from build123d import *

# Parameters (mm, degrees)
SKETCH1_R           = 25.5905
SKETCH1_R_2         = 19.2405
BOSS_EXTRUDE1_DEPTH = 7


with BuildPart() as part:
    # Sketch1 → Boss-Extrude1 (new body)
    with BuildSketch(Plane(origin=(0, 0, 0), x_dir=(1, 0, 0), z_dir=(0, 1, 0))):
        Circle(SKETCH1_R)
        Circle(SKETCH1_R_2, mode=Mode.SUBTRACT)
        Polygon((-12.131390351, -20.018099484), (13.231279228, -20.018099484), (13.231279228, -111.76), (38.036054145, -111.76), (38.036054145, -137.16), (-38.163945855, -137.16), (-38.163945855, -111.76), (-12.131390351, -111.76), align=None)
    extrude(amount=BOSS_EXTRUDE1_DEPTH)


solid = part.part
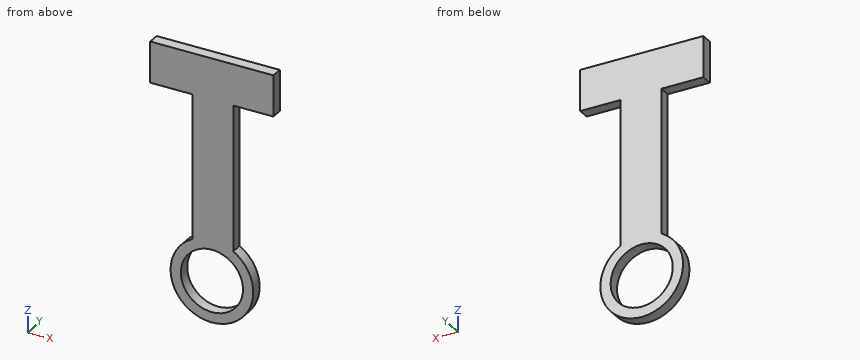
Can you work these out from the model? Positions are in its coordinate system, mm. Coordinates: 2 decimals unless noted, no trailing zeros. Loops run counter-clockwise (first coordinate to the right, second up) from the corner with the lowest first, then second, coordinate; pieces in that order, holes last. Notation, with made-up numbers: (27, 25.5) - (66, 25.5) arc R18 ccw to (66, 55.5) - close; hole circle Ø7 at (82.5, 44.25). An arc over 180 degrees is marked (long way). Put each result on its own line as item: value. Start each with the question number.
Item 1: If I drill on line 1 along Z through (x, y) = (0, 2.25); line 2 along X through (y, z) = (4.25, 0); line 3 along Z through (x, y) = (17.5, 1), over which ranges is the centre line in solid material (lowest first)?
Item 2: Suppose I cut it at D-D (z = 62). Please give me the cut outline in (x, y), and give its area (3 significant figures).
Item 3: For pin 1 (3.5 mm diameter, centred on y = 3, z = 86.5, fed in from +X); pin 2 (3.5 mm diameter, centred on x = -28, y = 3.5, fed in from -Z); pin 3 (1 mm diameter, centred on y = 1, z = -3.5, fed in from +X), each with a flat end and sliding along its axis, tell me the tip position at first contact or that it passes through.
Item 4: Suppose I cut it at B-B (x = 0). Please give me the cut outline in (y, z), and give its area (3 significant figures).
Item 5: Suppose I cut it at C-C (y = 5). Please give me the cut outline in (x, z), and give its area (3 significant figures).
Item 6: Suppose I cut it at A-A (z = 0). Please give me the cut outline in (x, y), and give its area (3 significant figures).
Here are the results:
1. line 1: -25.59 to -19.24, 19.24 to 137.16
1. line 2: -25.59 to -19.24, 19.24 to 25.59
1. line 3: -18.67 to -8, 8 to 18.67, 111.76 to 137.16
2. outline: (-12.13, 0) - (13.23, 0) - (13.23, 7) - (-12.13, 7) - close
2. area: 178 mm²
3. pin 1: x = 13.23
3. pin 2: z = 111.76
3. pin 3: x = 25.41
4. outline: (0, -25.59) - (7, -25.59) - (7, -19.24) - (0, -19.24) - close; (0, 19.24) - (7, 19.24) - (7, 137.16) - (0, 137.16) - close
4. area: 870 mm²
5. outline: (-38.16, 111.76) - (-12.13, 111.76) - (-12.13, 22.53) arc R25.59 ccw (long way) to (13.23, 21.9) - (13.23, 111.76) - (38.04, 111.76) - (38.04, 137.16) - (-38.16, 137.16) - close; hole circle Ø38.48 at (0, 0)
5. area: 5,040 mm²
6. outline: (-25.59, 0) - (-19.24, 0) - (-19.24, 7) - (-25.59, 7) - close; (19.24, 0) - (25.59, 0) - (25.59, 7) - (19.24, 7) - close
6. area: 88.9 mm²
